For this review, take the finished solid that the model builds, in its own axes (mm). Round coordinates to 2 decimals unless told otherwise and drop trailing zeros. Order: outer loops, then holes, each group sorted by start corner. A loop starts at its lowest first (then second) coordinate and runs counter-clockwise, first axis right, second up. Notation, with made-up numbers: (-9, 82) - (22, 82) arc R23 cw to (22, 99) - close; hole circle Ø1 at (-38.75, -35.5). An arc over 180 degrees is marked (long way). Write each question's results on one line, items separated by ' | '. Start each with the question number.
(1) Take a section at D-D, the plane z = 4. Give the boundary of the cut face in (x, y).
(2) Insertion check: pin 1 Ø8 at (x, z) = (67.5, -845.5) entering from +Y; pin 2 Ø5 at (x, z) = (66.5, 839.5) entering from +Y; pin 3 Ø4 at (x, z) = (69.5, -255.5) entering from +Y. Each pin has a flat end and moves straight along its axis. Give the tip position at first contact, or say it passes through.
(3) Take a section at A-A, the plane x = 2. Give the boundary of the cut face in (y, z), plus the area to 3 significant figures.
(4) Take a section at B-B, the plane y = 105.5. Give the boundary of the cut face in (x, z).
(5) Take a section at C-C, the plane z = 725. Give the boundary of the cut face in (x, y).
(6) For L1, parallel to X at y = 120, z = -588; L2, parallel to Y at x = -32.5, z = 606; L3, parallel to X at y = -57.5, z = -217, list the stretches that pass through material, from the lowest coordinate up. Write a range as from..to.
```python
from build123d import *

# Parameters (mm, degrees)
BOSS_EXTRUDE1_DEPTH                       = 925
CUT_EXTRUDE1_DEPTH                        = 30
FOR_MACH_SHOP_CONFIRM_W_PROGRAMMING_REACH = 951.777
SKETCH5_R                                 = 37.5
CUT_EXTRUDE3_DEPTH                        = 950.777089767
CUT_EXTRUDE4_REACH                        = 951.777
SKETCH6_R                                 = 25


with BuildPart() as part:
    # Sketch1 → Boss-Extrude1 (new, symmetric)
    with BuildSketch(Plane.XY):
        with BuildLine():
            Line((-50.8, -152.4), (50.8, -152.4))
            ThreePointArc((50.8, -152.4), (68.760512242, -144.960512242), (76.2, -127))
            Line((76.2, -127), (76.2, 127))
            ThreePointArc((76.2, 127), (68.760512242, 144.960512242), (50.8, 152.4))
            Line((50.8, 152.4), (-50.8, 152.4))
            ThreePointArc((-50.8, 152.4), (-68.760512242, 144.960512242), (-76.2, 127))
            Line((-76.2, 127), (-76.2, -127))
            ThreePointArc((-76.2, -127), (-68.760512242, -144.960512242), (-50.8, -152.4))
        make_face()
        with BuildLine():
            Line((-50.8, -139.7), (50.8, -139.7))
            ThreePointArc((50.8, -139.7), (59.780256121, -135.980256121), (63.5, -127))
            Line((63.5, -127), (63.5, 127))
            ThreePointArc((63.5, 127), (59.780256121, 135.980256121), (50.8, 139.7))
            Line((50.8, 139.7), (-50.8, 139.7))
            ThreePointArc((-50.8, 139.7), (-59.780256121, 135.980256121), (-63.5, 127))
            Line((-63.5, 127), (-63.5, -127))
            ThreePointArc((-63.5, -127), (-59.780256121, -135.980256121), (-50.8, -139.7))
        make_face(mode=Mode.SUBTRACT)
    extrude(amount=BOSS_EXTRUDE1_DEPTH, both=True)

    # Sketch2 → Cut-Extrude1 (cut)
    with BuildSketch(Plane(origin=(76.2, 0, 0), x_dir=(0, 0, -1), z_dir=(1, 0, 0))):
        with BuildLine():
            Line((-880, 37.6), (-825, 37.6))
            ThreePointArc((-825, 37.6), (-817.928932188, 34.671067812), (-815, 27.6))
            Line((-815, 27.6), (-815, -127.4))
            ThreePointArc((-815, -127.4), (-817.928932188, -134.471067812), (-825, -137.4))
            Line((-825, -137.4), (-880, -137.4))
            ThreePointArc((-880, -137.4), (-887.071067812, -134.471067812), (-890, -127.4))
            Line((-890, -127.4), (-890, 27.6))
            ThreePointArc((-890, 27.6), (-887.071067812, 34.671067812), (-880, 37.6))
        make_face()
        with BuildLine():
            Line((825, 37.6), (880, 37.6))
            ThreePointArc((880, 37.6), (887.071067812, 34.671067812), (890, 27.6))
            Line((890, 27.6), (890, -127.4))
            ThreePointArc((890, -127.4), (887.071067812, -134.471067812), (880, -137.4))
            Line((880, -137.4), (825, -137.4))
            ThreePointArc((825, -137.4), (817.928932188, -134.471067812), (815, -127.4))
            Line((815, -127.4), (815, 27.6))
            ThreePointArc((815, 27.6), (817.928932188, 34.671067812), (825, 37.6))
        make_face()
    extrude(amount=-CUT_EXTRUDE1_DEPTH, mode=Mode.SUBTRACT)

    # Sketch3 → for mach shop confirm w/ programming (cut, up to next)
    with BuildSketch(Plane(origin=(76.2, 0, 0), x_dir=(0, 0, -1), z_dir=(1, 0, 0)), mode=Mode.PRIVATE) as for_mach_shop_confirm_w_programming_sk1:
        with BuildLine():
            Line((-277.5, -45.65), (-222.5, -45.65))
            ThreePointArc((-222.5, -45.65), (-215.428932188, -48.578932188), (-212.5, -55.65))
            Line((-212.5, -55.65), (-212.5, -110.65))
            ThreePointArc((-212.5, -110.65), (-215.428932188, -117.721067812), (-222.5, -120.65))
            Line((-222.5, -120.65), (-277.5, -120.65))
            ThreePointArc((-277.5, -120.65), (-284.571067812, -117.721067812), (-287.5, -110.65))
            Line((-287.5, -110.65), (-287.5, -55.65))
            ThreePointArc((-287.5, -55.65), (-284.571067812, -48.578932188), (-277.5, -45.65))
        make_face()
    for_mach_shop_confirm_w_programming_tool1 = extrude(for_mach_shop_confirm_w_programming_sk1.sketch, amount=-FOR_MACH_SHOP_CONFIRM_W_PROGRAMMING_REACH, mode=Mode.PRIVATE) & part.part
    # Sketch3 → for mach shop confirm w/ programming (cut, up to next)
    with BuildSketch(Plane(origin=(76.2, 0, 0), x_dir=(0, 0, -1), z_dir=(1, 0, 0)), mode=Mode.PRIVATE) as for_mach_shop_confirm_w_programming_sk2:
        with BuildLine():
            Line((222.5, -45.65), (277.5, -45.65))
            ThreePointArc((277.5, -45.65), (284.571067812, -48.578932188), (287.5, -55.65))
            Line((287.5, -55.65), (287.5, -110.65))
            ThreePointArc((287.5, -110.65), (284.571067812, -117.721067812), (277.5, -120.65))
            Line((277.5, -120.65), (222.5, -120.65))
            ThreePointArc((222.5, -120.65), (215.428932188, -117.721067812), (212.5, -110.65))
            Line((212.5, -110.65), (212.5, -55.65))
            ThreePointArc((212.5, -55.65), (215.428932188, -48.578932188), (222.5, -45.65))
        make_face()
    for_mach_shop_confirm_w_programming_tool2 = extrude(for_mach_shop_confirm_w_programming_sk2.sketch, amount=-FOR_MACH_SHOP_CONFIRM_W_PROGRAMMING_REACH, mode=Mode.PRIVATE) & part.part
    add(for_mach_shop_confirm_w_programming_tool1.solids().sort_by_distance((76.2, -83.15, 250))[0], mode=Mode.SUBTRACT)
    add(for_mach_shop_confirm_w_programming_tool2.solids().sort_by_distance((76.2, -83.15, -250))[0], mode=Mode.SUBTRACT)

    # Sketch5 → Cut-Extrude3 (cut, through all)
    with BuildSketch(Plane.ZY.offset(76.2)):
        with Locations((725, 0)):
            Circle(SKETCH5_R)
        with Locations((-725, 0)):
            Circle(SKETCH5_R)
    extrude(amount=-CUT_EXTRUDE3_DEPTH, mode=Mode.SUBTRACT)

    # Sketch6 → Cut-Extrude4 (cut, up to next)
    with BuildSketch(Plane.ZY.offset(76.2), mode=Mode.PRIVATE) as cut_extrude4_sk1:
        with Locations((-375, 0)):
            Circle(SKETCH6_R)
    cut_extrude4_tool1 = extrude(cut_extrude4_sk1.sketch, amount=-CUT_EXTRUDE4_REACH, mode=Mode.PRIVATE) & part.part
    # Sketch6 → Cut-Extrude4 (cut, up to next)
    with BuildSketch(Plane.ZY.offset(76.2), mode=Mode.PRIVATE) as cut_extrude4_sk2:
        with Locations((300, 0)):
            Circle(SKETCH6_R)
    cut_extrude4_tool2 = extrude(cut_extrude4_sk2.sketch, amount=-CUT_EXTRUDE4_REACH, mode=Mode.PRIVATE) & part.part
    # Sketch6 → Cut-Extrude4 (cut, up to next)
    with BuildSketch(Plane.ZY.offset(76.2), mode=Mode.PRIVATE) as cut_extrude4_sk3:
        with Locations((425, 0)):
            Circle(SKETCH6_R)
    cut_extrude4_tool3 = extrude(cut_extrude4_sk3.sketch, amount=-CUT_EXTRUDE4_REACH, mode=Mode.PRIVATE) & part.part
    add(cut_extrude4_tool1.solids().sort_by_distance((-76.2, 0, -375))[0], mode=Mode.SUBTRACT)
    add(cut_extrude4_tool2.solids().sort_by_distance((-76.2, 0, 300))[0], mode=Mode.SUBTRACT)
    add(cut_extrude4_tool3.solids().sort_by_distance((-76.2, 0, 425))[0], mode=Mode.SUBTRACT)


solid = part.part
```
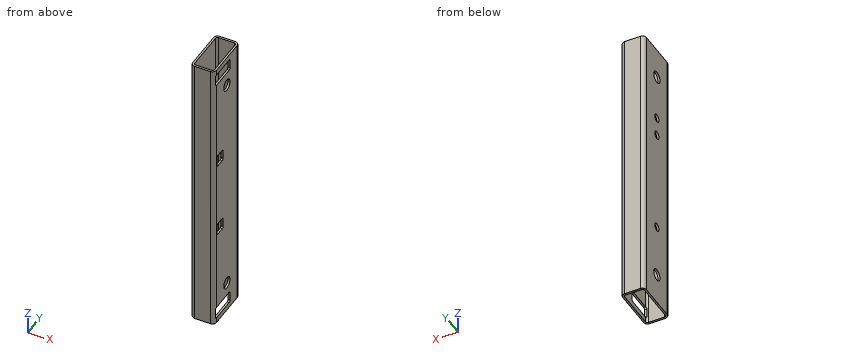
Results below:
1) outline: (-76.2, -127) arc R25.4 ccw to (-50.8, -152.4) - (50.8, -152.4) arc R25.4 ccw to (76.2, -127) - (76.2, 127) arc R25.4 ccw to (50.8, 152.4) - (-50.8, 152.4) arc R25.4 ccw to (-76.2, 127) - close; hole (-63.5, -127) arc R12.7 ccw to (-50.8, -139.7) - (50.8, -139.7) arc R12.7 ccw to (63.5, -127) - (63.5, 127) arc R12.7 ccw to (50.8, 139.7) - (-50.8, 139.7) arc R12.7 ccw to (-63.5, 127) - close
2) pin 1: stops at y = 149 | pin 2: stops at y = 148.7 | pin 3: stops at y = 146.14
3) outline: (-152.4, -925) - (-139.7, -925) - (-139.7, 925) - (-152.4, 925) - close; (139.7, -925) - (152.4, -925) - (152.4, 925) - (139.7, 925) - close | area: 47,000 mm^2
4) outline: (-76.2, -925) - (-63.5, -925) - (-63.5, 925) - (-76.2, 925) - close; (63.5, -925) - (76.2, -925) - (76.2, 925) - (63.5, 925) - close
5) outline: (-76.2, -127) arc R25.4 ccw to (-50.8, -152.4) - (50.8, -152.4) arc R25.4 ccw to (76.2, -127) - (76.2, -37.5) - (63.5, -37.5) - (63.5, -127) arc R12.7 cw to (50.8, -139.7) - (-50.8, -139.7) arc R12.7 cw to (-63.5, -127) - (-63.5, -37.5) - (-76.2, -37.5) - close; (-76.2, 37.5) - (-63.5, 37.5) - (-63.5, 127) arc R12.7 cw to (-50.8, 139.7) - (50.8, 139.7) arc R12.7 cw to (63.5, 127) - (63.5, 37.5) - (76.2, 37.5) - (76.2, 127) arc R25.4 ccw to (50.8, 152.4) - (-50.8, 152.4) arc R25.4 ccw to (-76.2, 127) - close
6) L1: x = -76.2..-63.5, 63.5..76.2 | L2: y = -152.4..-139.7, 139.7..152.4 | L3: x = -76.2..-63.5
